Part model, mm, in its own coordinate system. Round coordinates to 2 decimals unless told otherwise and drop trailing zeros. Write each loop counter-clockwise with the first axis right and the second up, starting at its lowest first coordinate (ties: lowest second). Pieces come first, ordered by that corner, then holes.
Autodesk Inventor part; units mm, degrees
ref_plane "YZ Plane" through (0, 0, 0) normal (1, 0, 0) x (0, 1, 0)
ref_plane "XZ Plane" through (0, 0, 0) normal (0, 1, 0) x (-1, 0, 0)
ref_plane "XY Plane" through (0, 0, 0) normal (0, 0, 1) x (1, 0, 0)
sketch "Sketch1" plane through (0, 0, 0) normal (0, 1, 0) x (-1, 0, 0)
  line L0 (-3.175, 3.175) -> (3.175, 3.175)
  line L1 (3.175, 3.175) -> (3.175, -3.175)
  line L2 (3.175, -3.175) -> (-3.175, -3.175)
  line L3 (-3.175, -3.175) -> (-3.175, 3.175)
  line L4 (-3.175, 3.175) -> (3.175, -3.175) construction
  line L5 (3.175, 3.175) -> (-3.175, -3.175) construction
  point P0 (0, 0)
  dimension "d0" = 6.35
  dimension "d1" = 6.35
extrude "Extrusion1" add sketch "Sketch1" along normal blind 228.6
fillet "Fillet1" radius 1.5875 4 edges at (3.175, 114.3, -3.175) (3.175, 114.3, 3.175) (-3.175, 114.3, 3.175) (-3.175, 114.3, -3.175)
fillet "Fillet2" radius 0.7937 16 edges at (3.175, 0, 0) (2.71, 0, -2.71) (0, 0, -3.175) (-2.71, 0, -2.71) (-3.175, 0, 0) (-2.71, 0, 2.71) (0, 0, 3.175) (2.71, 0, 2.71) (0, 228.6, 3.175) (-2.71, 228.6, 2.71) (-3.175, 228.6, 0) (-2.71, 228.6, -2.71) (0, 228.6, -3.175) (2.71, 228.6, -2.71) (3.175, 228.6, 0) (2.71, 228.6, 2.71)
properties part number "9 inch hs shaft" material "Stainless Steel"
Q1. Wall check: L1, parallel to Z at x = -1.75, y = 57.5; L2, parallel to Y at x = -1.5, z = 2.5; L3, parallel to Z at x = -2.25, y = 94. Give the ranges that are in metal, low to high.
Values follow:
L1: z = -3.17 to 3.17
L2: y = 0.01 to 228.59
L3: z = -3.03 to 3.03
Q2. Drop a flat-ended pin along its axis: pin 1 (2 mm diameter, centred on x = 2.5, y = 104, fed in from +Z) (3 decimals). Give the stop position or say it passes through.
Values follow:
pin 1: stops at z = 3.175
Q3. Cut at A-A on y = 68. Write the cut outline in (x, z) (1 decimal), plus the area to 3 significant figures.
Values follow:
outline: (-3.2, -1.6) arc R1.6 ccw to (-1.6, -3.2) - (1.6, -3.2) arc R1.6 ccw to (3.2, -1.6) - (3.2, 1.6) arc R1.6 ccw to (1.6, 3.2) - (-1.6, 3.2) arc R1.6 ccw to (-3.2, 1.6) - close
area: 38.2 mm2
